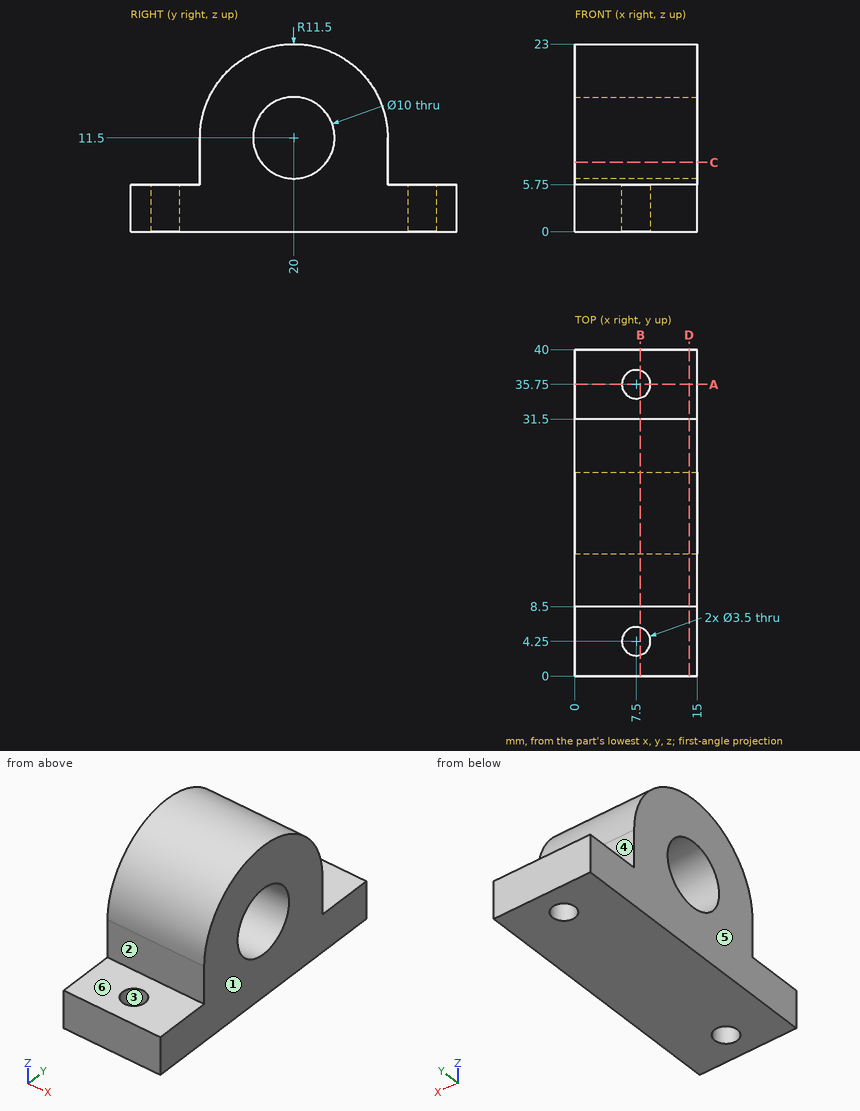
Source: three-view drawing plus pictorial views. Frame: mm from the lowest corner of the part. A direction names the side the tool comes from. Coordinates: 2 decimals unless noted, no trailing zeros. Order: outer loops, then holes, each group sorted by start corner. A loop starts at its lowest first (then second) coordinate and runs counter-clockwise, first axis right, second up.
Item 1: Cut plane B-B (x = 8). Return loops of the section in (y, z).
Output values:
outline: (0, 0) - (2.57, 0) - (2.57, 5.75) - (0, 5.75) - close; (5.93, 0) - (34.07, 0) - (34.07, 5.75) - (31.5, 5.75) - (31.5, 11.5) arc R11.5 ccw to (8.5, 11.5) - (8.5, 5.75) - (5.93, 5.75) - close; (37.43, 0) - (40, 0) - (40, 5.75) - (37.43, 5.75) - close; hole circle Ø10 at (20, 11.5)
Item 2: First-contact query: P1, Ø5.5, axis at x = 7.5, y = 4.25, coming from the +Z side; P2, Ø12, axis at y = 27.5, z = 15.5, coming from the -X side; P3, Ø6, axis at x = 5.5, y = 6.5, coming from the +Z side; P4, Ø3, axis at x = 10.5, z = 15, coming from the -Y side. Flat tips, straight axial feed; report the tip coordinate or a pass-through.
Output values:
P1: stops at z = 5.75
P2: stops at x = 0
P3: stops at z = 16.19
P4: stops at y = 8.68
Item 3: Pull-direction query (Y, two-part tool) for the marked faces 1, 2 and 3; classes: pulls with the +Y half, pulls with the -Y half, needs draft (parallel to the pull), parting line crosses it, or undercut.
Output values:
face 1: needs draft
face 2: pulls with the -Y half
face 3: undercut
Item 4: Cut plane D-D (x = 14). Return loops of the section in (y, z), plus the area to 3 significant figures.
Output values:
outline: (0, 0) - (40, 0) - (40, 5.75) - (31.5, 5.75) - (31.5, 11.5) arc R11.5 ccw to (8.5, 11.5) - (8.5, 5.75) - (0, 5.75) - close; hole circle Ø10 at (20, 11.5)
area: 491 mm2
Item 5: Set-up query: the marked faces 4, 5 and 6. Return all of +Z, -Z, +X, -X, +Y, -Y with unobstructed straight access to the full face (end or side cutting, diameter ignored); none if empty.
Output values:
face 4: +Z, +X, -X, +Y
face 5: +Z, -Z, -X, +Y, -Y
face 6: +Z, +X, -X, -Y
Item 6: Cut plane A-A (y = 35.75). Return loops of the section in (x, z), plus the area to 3 significant figures.
Output values:
outline: (0, 0) - (5.75, 0) - (5.75, 5.75) - (0, 5.75) - close; (9.25, 0) - (15, 0) - (15, 5.75) - (9.25, 5.75) - close
area: 66.1 mm2
Item 7: Material intervals for line 1 (Y direction, x = 7.5, z = 3.35); line 2 (X direction, y = 4.25, z = 2.75); line 3 (Y direction, x = 7, z = 1.5), sorted ascending.
Output values:
line 1: y = 0 to 2.5, 6 to 34, 37.5 to 40
line 2: x = 0 to 5.75, 9.25 to 15
line 3: y = 0 to 2.57, 5.93 to 34.07, 37.43 to 40
Item 8: Cut plane C-C (z = 8.5). Return loops of the section in (x, y).
Output values:
outline: (0, 8.5) - (15, 8.5) - (15, 16) - (0, 16) - close; (0, 24) - (15, 24) - (15, 31.5) - (0, 31.5) - close
